The drawing under review shows one solid part. Ordinate dimensions are in mm from its lowest x, y, z. A direction names the side the tool comes from. Coordinates: 2 decimals unless noted, no trailing zeros. Write each loop counter-clockwise with the first axis right and the second up, starting at its lowest first coordinate (ties: lowest second). Pieces come first, ordered by that corner, then holes. Notation, with made-up numbers: (62, 22.25) - (116, 22.25) arc R12 cw to (116, 35.25) - close; hole circle Ø1 at (44.5, -12). An arc over 180 degrees is marked (long way). Put each result on its own line as item: value. Start each with the question number.
Item 1: Machinability: for the marked faces 1 and 2, which of the approach directions +Z, -Z, +X, -X, +Y, -Y give a long, thin tool a straight path to every point of the face, cutting with its end or side? Answer none if there is none.
Item 2: Consider section B-B on z = 6.5. Give the boundary of the cut face in (x, y), then the cut area to 3 significant figures.
Item 3: Consider section A-A on x = 90.5. Give the boundary of the cut face in (y, z), then the cut area to 4 significant figures.
Item 4: To check wall thickness, follow L1, parallel to Y at x = 96, z = 15.5; L2, parallel to X at y = 24, z = 31 (1 decimal); L3, parallel to X at y = 15.5, z = 59.5 (1 decimal). State the ranges of each line that lie inside material, in increasing order. Write a range as [from, to].
Item 5: For pin 1 (12 mm diameter, centred on x = 104.5, z = 64, fed in from -Y); pin 2 (4 mm diameter, centred on y = 5, z = 43, fed in from -X); pin 3 (10 mm diameter, centred on x = 25, y = 21, fed in from +Z), all flat-tipped, find the tip position at first contact; note any pin that passes through.
Item 6: Consider section C-C on y = 23. Give the boundary of the cut face in (x, z).
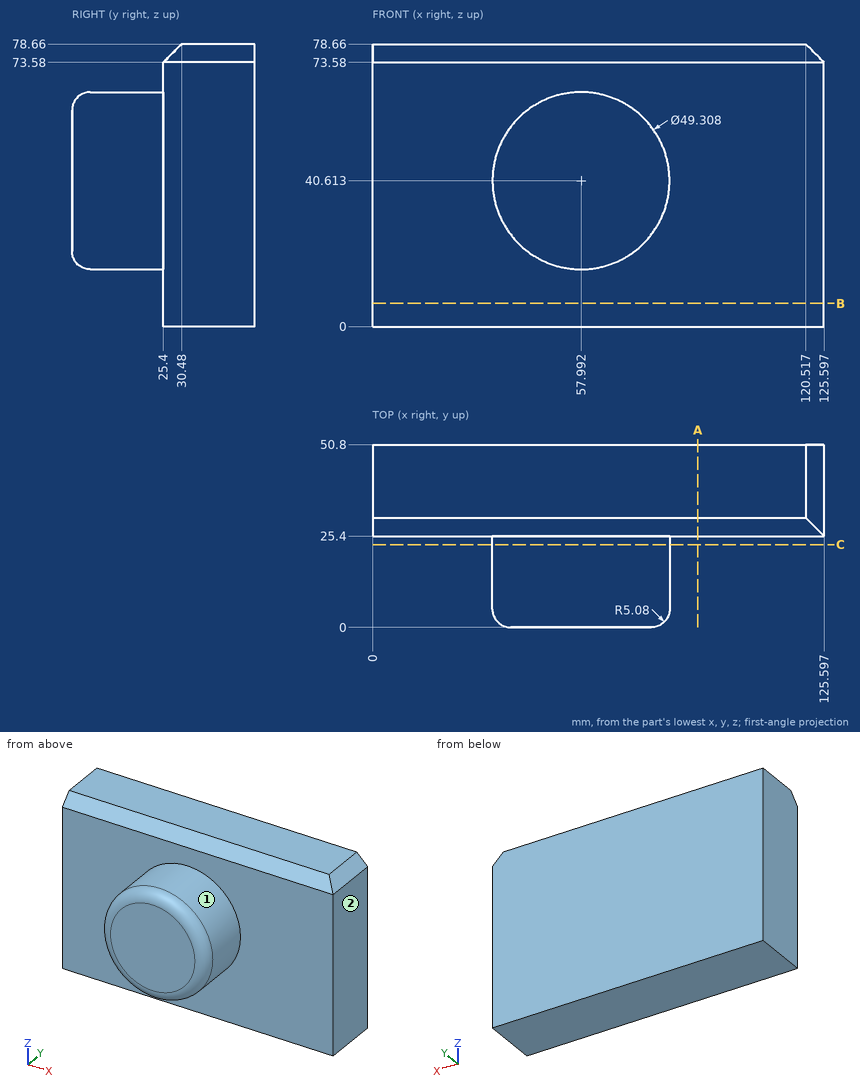
Report:
1. face 1: -Y
1. face 2: +Z, -Z, +X, +Y, -Y
2. outline: (0, 25.4) - (125.6, 25.4) - (125.6, 50.8) - (0, 50.8) - close
2. area: 3,190 mm²
3. outline: (25.4, 0) - (50.8, 0) - (50.8, 78.66) - (30.48, 78.66) - (25.4, 73.58) - close
3. area: 1,985 mm²
4. L1: [25.4, 50.8]
4. L2: [35.3, 80.7]
4. L3: [42.1, 73.8]
5. pin 1: y = 25.4
5. pin 2: x = 33.34
5. pin 3: z = 74.18
6. outline: circle Ø49.31 at (57.99, 40.61)
